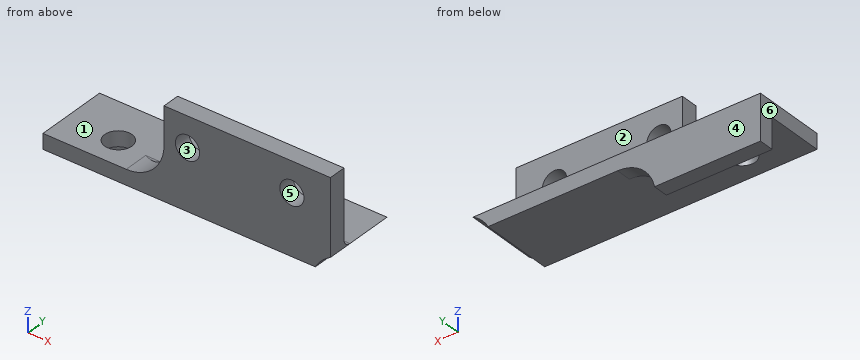
from build123d import *

# Parameters (mm, degrees)
CROQUIS1_W              = 2
CROQUIS1_H              = 2
CROQUIS1_W_2            = 4
SALIENTE_EXTRUIR1_DEPTH = 14
CROQUIS1_3_W            = 2
CROQUIS1_3_H            = 2
SALIENTE_EXTRUIR2_DEPTH = 22
CORTAR_EXTRUIR1_DEPTH   = 2
CROQUIS2_3_W            = 18
CROQUIS2_3_H            = 2.3
CROQUIS2_3_W_2          = 2
SALIENTE_EXTRUIR3_DEPTH = 10
CROQUIS3_R              = 1.6
CORTAR_EXTRUIR2_DEPTH   = 2.3
REDONDEO1_R             = 5
REDONDEO4_START         = -3.8
REDONDEO4_DEPTH         = 9.6
REDONDEO5_R             = 1
REDONDEO6_R             = 5


with BuildPart() as part:
    # Croquis1 → Saliente-Extruir1 (new body)
    with BuildSketch(Plane(origin=(0, 0, 0), x_dir=(0, 0, -1), z_dir=(1, 0, 0))):
        Polygon((0, -3.8), (0, 0), (0, 3.8), (-2, 3.8), (-2, -3.8), align=None)
        with Locations((-1, 4.8)):
            Rectangle(CROQUIS1_W, CROQUIS1_H)
        with Locations((2, 4.8)):
            Rectangle(CROQUIS1_W_2, CROQUIS1_H)
    extrude(amount=-SALIENTE_EXTRUIR1_DEPTH)

    # Croquis1<3> → Saliente-Extruir2 (add)
    with BuildSketch(Plane(origin=(0, 0, 0), x_dir=(0, 0, -1), z_dir=(1, 0, 0))):
        Polygon((0, -3.8), (0, 0), (0, 3.8), (-2, 3.8), (-2, -3.8), align=None)
        with Locations((-1, 4.8)):
            Rectangle(CROQUIS1_3_W, CROQUIS1_3_H)
    extrude(amount=SALIENTE_EXTRUIR2_DEPTH)

    # Croquis2 → Cortar-Extruir1 (cut)
    with BuildSketch(Plane.XY.offset(2)):
        with BuildLine():
            ThreePointArc((-8.8, 0), (-7, -1.8), (-5.2, 0))
            Line((-5.2, 0), (-8.8, 0))
        make_face()
        with BuildLine():
            Line((-8.8, 0), (-5.2, 0))
            ThreePointArc((-5.2, 0), (-7, 1.8), (-8.8, 0))
        make_face()
    extrude(amount=-CORTAR_EXTRUIR1_DEPTH, mode=Mode.SUBTRACT)

    # Croquis2<3> → Saliente-Extruir3 (add)
    with BuildSketch(Plane.XY.offset(2)):
        with Locations((13, -2.65)):
            Rectangle(CROQUIS2_3_W, CROQUIS2_3_H)
        with Locations((3, -2.65)):
            Rectangle(CROQUIS2_3_W_2, CROQUIS2_3_H)
        with Locations((23, -2.65)):
            Rectangle(CROQUIS2_3_W_2, CROQUIS2_3_H)
    extrude(amount=SALIENTE_EXTRUIR3_DEPTH)

    # Croquis3 → Cortar-Extruir2 (cut)
    with BuildSketch(Plane(origin=(0, -1.5, 0), x_dir=(1, 0, 0), z_dir=(0, 1, 0))):
        with Locations(Location((5.1, -8, 0), (0, 0, 180))):
            Circle(CROQUIS3_R)
        with Locations(Location((18.9, -8, 0), (0, 0, 180))):
            Circle(CROQUIS3_R)
    extrude(amount=-CORTAR_EXTRUIR2_DEPTH, mode=Mode.SUBTRACT)

    # Redondeo1
    # the kernel refuses this fillet: 5 mm, written as the material it adds along each edge
    with BuildSketch(Plane(origin=(0, 3.8, 0), x_dir=(1, 0, 0), z_dir=(0, 1, 0))) as redondeo1_piece_1:
        with BuildLine():
            CenterArc((4.898979486, 5), REDONDEO1_R, 191.536959033, 78.463040967)
            Line((0, 4), (-0.09797959, 3.98))
            ThreePointArc((-0.09797959, 3.98), (-0.1, 2), (-0.1, 0))
            Line((-0.1, 0), (0, -0.1))
            Line((0, -0.1), (4.898979486, -0.1))
            Line((4.898979486, -0.1), (4.898979486, 0))
        make_face()
    extrude(amount=2)

    # Redondeo4: read off the stored shape, not the designer's step
    # Redondeo4 outline → Redondeo4 (add)
    with BuildSketch(Plane(origin=(0, 0, 0), x_dir=(1, 0, 0), z_dir=(0, 1, 0)).offset(REDONDEO4_START)):
        with BuildLine():
            ThreePointArc((24, -2), (22.855631086, -1.144368914), (22, 0))
            Line((22, 0), (22, -2))
            Line((22, -2), (24, -2))
        make_face()
    extrude(amount=REDONDEO4_DEPTH)

    # Redondeo5
    redondeo5_edges = [part.edges().sort_by_distance(p)[0] for p in [
        (13, -1.5, 2),
    ]]
    fillet(redondeo5_edges, radius=REDONDEO5_R)

    # Redondeo6
    redondeo6_edges = [part.edges().sort_by_distance(p)[0] for p in [
        (2, -2.15, 2),
    ]]
    fillet(redondeo6_edges, radius=REDONDEO6_R)


solid = part.part
Geometry: final body of the model. Coordinates: model frame, mm. Face numbers are marked on the shaded views. A direction names the side the tool comes from. Give positions to 0.01 mm unless a question says otherwise; leave off trailing zeros. Write each loop counter-clockwise with the first axis right and the second up, starting at its lowest first coordinate (ties: lowest second). Pieces come first, ordered by that corner, then holes. Notation, with made-up numbers: (63.25, 65.25) -> (102.25, 65.25) arc R27 cw to (102.25, 96.25) -> close; hole circle Ø6 at (-18, 71.25). An arc over 180 degrees is marked (long way). Answer as a JSON object with one key per item and string values.
1. Cut plane A-A on x = -7. Output: boundary loops of the cut face in (y, z), and give its area (3 significant figures).
Ans:
{"outline": "(-3.8, 0) -> (-1.8, 0) -> (-1.8, 2) -> (-3.8, 2) -> close; (1.8, 0) -> (3.8, 0) -> (3.8, -4) -> (5.8, -4) -> (5.8, 2) -> (1.8, 2) -> close", "area": "20.0 mm^2"}
2. Contact query for flat-ended pins moving along their axis: pin 1 (5 mm diameter, centred on x = 7.5, y = 3, fed in from -Z); pin 2 (3.5 mm diameter, centred on x = 18.9, z = 8, fed in from -Y); pin 3 (2 mm diameter, centred on x = -3.5, z = -2, fed in from -Y); pin 4 (2.5 mm diameter, centred on x = 13, z = 9, fed in from +Y). Output: stop coordinate, or through.
Ans:
{"pin 1": "stops at z = 0", "pin 2": "stops at y = -3.8", "pin 3": "stops at y = 3.8", "pin 4": "stops at y = -1.5"}
3. Access query for the marked faces 1, 2 and 3. Directions: +Z, -Z, +X, -X, +Y, -Y. A direction counts if a zero-diameter tool reaches every point of the face in a straight line with its end or side. Return the directions, or none.
Ans:
{"face 1": "+Z, -X, +Y", "face 2": "+Z, +X, -X, +Y", "face 3": "+Y, -Y"}
4. Ray query, probe 1 along Y at (x, z) = (-7, 1); probe 2 along Z at (x, y) = (-9.5, 4.75); probe 3 along Z at (x, y) = (11, 5.5). Return the intervals inside material, ascending. Write a range as from..to.
Ans:
{"probe 1": "y = -3.8..-1.8, 1.8..5.8", "probe 2": "z = -4..2", "probe 3": "z = 0..2"}
5. Cut plane C-C on y = 0. Output: boundary loops of the cut face in (x, z), and give its area (3 significant figures).
Ans:
{"outline": "(-14, 0) -> (-8.8, 0) -> (-8.8, 2) -> (-14, 2) -> close; (-5.2, 0) -> (22, 0) arc R5 cw to (24, 2) -> (-5.2, 2) -> close", "area": "66.4 mm^2"}
6. Mould query, pull axis X, two halves, no side actions, for the marked faces 4, 5 and 6. Classes: pulls with the +X half, pulls with the -X half, needs draft (parallel to the pull), parting line crosses it, or undercut.
Ans:
{"face 4": "needs draft", "face 5": "undercut", "face 6": "pulls with the -X half"}
7. Cut plane D-D on y = -2.5. Output: boundary loops of the cut face in (x, z), and give its area (3 significant figures).
Ans:
{"outline": "(-14, 0) -> (22, 0) arc R5 cw to (24, 2) -> (24, 12) -> (2, 12) -> (2, 7) arc R5 cw to (-3, 2) -> (-14, 2) -> close; hole circle Ø3.2 at (5.1, 8); hole circle Ø3.2 at (18.9, 8)", "area": "283 mm^2"}
8. Cut plane B-B on z = 8. Output: boundary loops of the cut face in (x, y), and give its area (3 significant figures).
Ans:
{"outline": "(2, -3.8) -> (3.5, -3.8) -> (3.5, -1.5) -> (2, -1.5) -> close; (6.7, -3.8) -> (17.3, -3.8) -> (17.3, -1.5) -> (6.7, -1.5) -> close; (20.5, -3.8) -> (24, -3.8) -> (24, -1.5) -> (20.5, -1.5) -> close", "area": "35.9 mm^2"}
